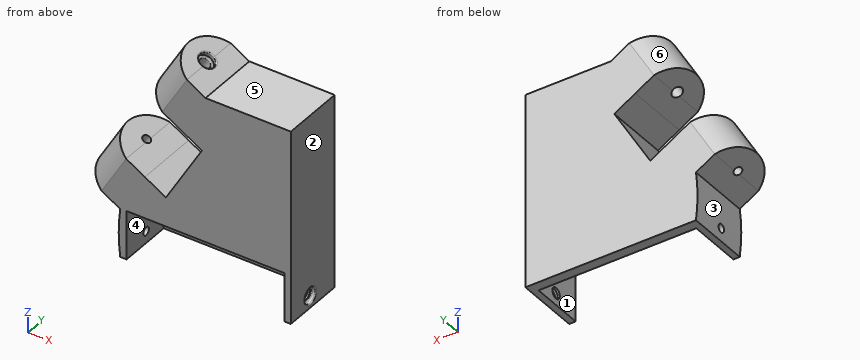
```python
from build123d import *

# Parameters (mm, degrees)
BOSS_EXTRUDE2_DEPTH                             = 29.972
EXTRUDE_THIN2_DEPTH                             = 29.972
BOSS_EXTRUDE3_DEPTH                             = 22.86
BOSS_EXTRUDE4_DEPTH                             = 22.86
SKETCH12_R                                      = 1.905
CUT_EXTRUDE2_DEPTH                              = 111.410659875
BOSS_EXTRUDE6_DEPTH                             = 29.972
CBORE_FOR_6_PAN_HEAD_MACHINE_SCREW1_D           = 3.7500052
CBORE_FOR_6_PAN_HEAD_MACHINE_SCREW1_CBORE_D     = 7.5000104
CBORE_FOR_6_PAN_HEAD_MACHINE_SCREW1_CBORE_DEPTH = 2.032
CUT_EXTRUDE4_REACH                              = 107.839
SKETCH18_R                                      = 2.5
FILLET1_R                                       = 0.5
SKETCH19_W                                      = 73.969126852
SKETCH19_H                                      = 25.4
CUT_EXTRUDE5_DEPTH                              = 22.86
CUT_EXTRUDE7_START                              = -80.649491
SKETCH21_R                                      = 1.905
CUT_EXTRUDE7_DEPTH                              = 80.649491
CBORE_FOR_6_PAN_HEAD_MACHINE_SCREW2_D           = 3.7500052
CBORE_FOR_6_PAN_HEAD_MACHINE_SCREW2_CBORE_D     = 7.5000104
CBORE_FOR_6_PAN_HEAD_MACHINE_SCREW2_CBORE_DEPTH = 2.032
SKETCH26_R                                      = 2.54
CUT_EXTRUDE9_DEPTH                              = 3.048
FILLET3_R                                       = 0.5
CUT_EXTRUDE11_DEPTH                             = 29.972


with BuildPart() as part:
    # Sketch1 → Boss-Extrude2 (new body)
    with BuildSketch(Plane(origin=(0, 0, 0), x_dir=(1, 0, 0), z_dir=(0, 1, 0))):
        Polygon((-40.005, 45.466), (-40.005, 22.86), (0, -45.466), (40.005, -45.466), (40.005, 45.466), align=None)
    extrude(amount=BOSS_EXTRUDE2_DEPTH)

    # Sketch8 → Extrude-Thin2 (add)
    with BuildSketch(Plane(origin=(0, 0, 0), x_dir=(1, 0, 0), z_dir=(0, 1, 0))):
        Polygon((-40.005, 22.86), (-28.454605215, 3.132659066), (-37.222312297, -2.000849727), (-48.772707082, 17.726491207), align=None)
        Polygon((-11.550394785, -25.738659066), (0, -45.466), (-8.767707082, -50.599508793), (-20.318101866, -30.872167859), align=None)
    extrude(amount=EXTRUDE_THIN2_DEPTH)

    # Sketch10 → Boss-Extrude3 (add)
    with BuildSketch(Plane(origin=(19.824382752, 0, 33.85878705), x_dir=(0.862963295, 0, -0.505266614), z_dir=(0.505266614, 0, 0.862963295))):
        with BuildLine():
            Line((-33.132451849, 29.972), (-33.132451849, 0))
            ThreePointArc((-33.132451849, 0), (-44.041101893, 14.986), (-33.132451849, 29.972))
        make_face()
    extrude(amount=-BOSS_EXTRUDE3_DEPTH)

    # Sketch11 → Boss-Extrude4 (add)
    with BuildSketch(Plane(origin=(-8.630222463, 0, -14.739872016), x_dir=(0.862963295, 0, -0.505266614), z_dir=(0.505266614, 0, 0.862963295))):
        with BuildLine():
            Line((-33.132451849, 0), (-33.132451849, 29.972))
            ThreePointArc((-33.132451849, 29.972), (-44.041101893, 14.986), (-33.132451849, 0))
        make_face()
    extrude(amount=-BOSS_EXTRUDE4_DEPTH)

    # Sketch12 → Cut-Extrude2 (cut, through all)
    with BuildSketch(Plane(origin=(21.107759951, 0, 36.050713821), x_dir=(0.862963295, 0, -0.505266614), z_dir=(0.505266614, 0, 0.862963295))):
        with Locations((-33.881101893, 14.986)):
            Circle(SKETCH12_R)
    extrude(amount=-CUT_EXTRUDE2_DEPTH, mode=Mode.SUBTRACT)

    # Sketch15 → Boss-Extrude6 (add)
    with BuildSketch(Plane(origin=(0, 29.972, 0), x_dir=(1, 0, 0), z_dir=(0, 1, 0))):
        with BuildLine():
            Line((-40.005, 45.466), (-40.005, 22.86))
            ThreePointArc((-40.005, 22.86), (-40.726132774, 34.163), (-40.005, 45.466))
        make_face()
    extrude(amount=-BOSS_EXTRUDE6_DEPTH)

    # CBORE for #6 Pan Head Machine Screw1 (through all)
    with Locations(Plane(origin=(19.824382752, 0, 33.85878705), x_dir=(0.862963295, 0, -0.505266614), z_dir=(0.505266614, 0, 0.862963295))):
        with Locations((-33.881101893, 14.986)):
            CounterBoreHole(CBORE_FOR_6_PAN_HEAD_MACHINE_SCREW1_D / 2, CBORE_FOR_6_PAN_HEAD_MACHINE_SCREW1_CBORE_D / 2, CBORE_FOR_6_PAN_HEAD_MACHINE_SCREW1_CBORE_DEPTH)

    # Sketch18 → Cut-Extrude4 (cut, up to next)
    with BuildSketch(Plane(origin=(18.797680994, 0, 32.105245634), x_dir=(0.862963295, 0, -0.505266614), z_dir=(0.505266614, 0, 0.862963295)), mode=Mode.PRIVATE) as cut_extrude4_sk1:
        with Locations((-33.881101893, 14.986)):
            Circle(SKETCH18_R)
    cut_extrude4_tool1 = extrude(cut_extrude4_sk1.sketch, amount=-CUT_EXTRUDE4_REACH, mode=Mode.PRIVATE) & part.part
    add(cut_extrude4_tool1.solids().sort_by_distance((-10.440466, 14.986, 49.224235))[0], mode=Mode.SUBTRACT)

    # Fillet1
    fillet1_edges = [part.edges().sort_by_distance(p)[0] for p in [
        (-12.649881436, 14.986, 52.872529093),
        (-12.597874588, 14.986, 50.487401783),
    ]]
    fillet(fillet1_edges, radius=FILLET1_R)

    # Sketch19 → Cut-Extrude5 (cut)
    with BuildSketch(Plane(origin=(0, 0, -45.466), x_dir=(-1, 0, 0), z_dir=(0, 0, -1))):
        with Locations((0.027563426, 12.7)):
            Rectangle(SKETCH19_W, SKETCH19_H)
    extrude(amount=-CUT_EXTRUDE5_DEPTH, mode=Mode.SUBTRACT)

    # Sketch21 → Cut-Extrude7 (cut)
    with BuildSketch(Plane(origin=(40.005, 0, 0), x_dir=(0, 0, -1), z_dir=(1, 0, 0)).offset(CUT_EXTRUDE7_START)):
        with Locations((39.878, 13.391837379)):
            Circle(SKETCH21_R)
    extrude(amount=CUT_EXTRUDE7_DEPTH, mode=Mode.SUBTRACT)

    # CBORE for #6 Pan Head Machine Screw2 (through all)
    with Locations(Plane(origin=(40.005, 0, 0), x_dir=(0, 0, -1), z_dir=(1, 0, 0))):
        with Locations((39.878, 13.391837379)):
            CounterBoreHole(CBORE_FOR_6_PAN_HEAD_MACHINE_SCREW2_D / 2, CBORE_FOR_6_PAN_HEAD_MACHINE_SCREW2_CBORE_D / 2, CBORE_FOR_6_PAN_HEAD_MACHINE_SCREW2_CBORE_DEPTH)

    # Sketch26 → Cut-Extrude9 (cut)
    with BuildSketch(Plane(origin=(40.005, 0, 0), x_dir=(0, 0, -1), z_dir=(1, 0, 0))):
        with Locations(Location((39.878, 13.391837379, 0), (0, 0, 180))):  # turned: the seam where the file's is
            Circle(SKETCH26_R)
    extrude(amount=-CUT_EXTRUDE9_DEPTH, mode=Mode.SUBTRACT)

    # Fillet3
    fillet3_edges = [part.edges().sort_by_distance(p)[0] for p in [
        (40.005, 13.391837379, -36.1279948),
        (37.973, 13.391837379, -36.1279948),
    ]]
    fillet(fillet3_edges, radius=FILLET3_R)

    # Sketch28 → Cut-Extrude11 (cut)
    with BuildSketch(Plane(origin=(0, 29.972, 0), x_dir=(1, 0, 0), z_dir=(0, 1, 0))):
        Polygon((-11.550394785, -25.738659066), (-1.686724318, -19.963461674), (-18.590934748, 8.907856459), (-28.454605215, 3.132659066), align=None)
    extrude(amount=-CUT_EXTRUDE11_DEPTH, mode=Mode.SUBTRACT)


solid = part.part
```
The listing builds one solid part. Answer for the finished solid, in the listing's coordinates (mm). Face numbers are marked on the shaded views. A direction names the side the tool comes from. Give positions to 0.01 mm unless a question says otherwise; leave off trailing zeros. Order: outer loops, then holes, each group sorted by start corner. A loop starts at its lowest first (then second) coordinate and runs counter-clockwise, first axis right, second up. Notation, with made-up numbers: (78.5, 55.25) -> (96.5, 55.25) arc R30 ccw to (96.5, 84.25) -> close; hole circle Ø10 at (18.25, 1). An arc over 180 degrees is marked (long way). Answer as a JSON object with one key per item and string values. Group by question number.
Item 1: The part is cut by section C-C on y = 6.75. Write down the section's boundary in (x, z) (1 decimal), and give its area (3 significant figures).
Item 2: Flat-ended cylindrical pins translate along their axes: pin 1 (5 mm diameter, centred on y = 13.39, z = -39.88, fed in from +X); pin 2 (7 mm diameter, centred on y = 14, z = -40, fed in from +X); pin 3 (10 mm diameter, centred on y = 13.39, z = -39.88, fed in from -X). Find the tip coordinate at first contact, or state that the pin passes through.
Item 3: Consider L1, parallel to X at y = 24.5, z = -37.5 (3 decimals); L2, parallel to Z at x = 23, y = 7.25; L3, parallel to Y at x = 0.5, z = -38. Determine where each line is inside the solid, lowest interval first. Write a range as from..to.
Item 4: The part is cut by section B-B on z = -25. Write down the section's boundary in (x, y) (3 decimals), and give its area (3 significant figures).
Item 5: Determine the mould class of the marked faces 1, 2 and 3 for opening direction X: pulls with the +X half, pulls with the -X half, needs draft (parallel to the pull), parting line crosses it, or undercut.
Item 6: A tool of negligible diameter and unlimited length cuts with its end or side. For the marked faces 4, 5 and 6, from which of +Z, -Z, +X, -X, +Y, -Y can it reach the whole face along a straight path? Write none if from no direction.
Item 7: The part is cut by section A-A on x = 15. Write down the section's boundary in (y, z).
Item 8: The part is cut by section D-D on y = 23. Write down the section's boundary in (x, z) (1 decimal), and give its area (3 significant figures).
Result set:
{
 "1": {"outline": "(-56.2, -13.4) -> (-40, -22.9) arc R88.9 ccw to (-40, -45.5) -> (-37, -45.5) -> (-37, -22.6) -> (37, -22.6) -> (37, -45.5) -> (40, -45.5) -> (40, 45.5) -> (0, 45.5) -> (-16.2, 54.9) -> (-27.7, 35.2) -> (-1.7, 20) -> (-18.6, -8.9) -> (-44.6, 6.3) -> close", "area": "4,700 mm²"},
 "2": {"pin 1": "x = -37.01", "pin 2": "x = 39.99", "pin 3": "x = -40.72"},
 "3": {"L1": "-40.664..-37.012, 36.957..40.005", "L2": "-22.61..45.47", "L3": "25.4..29.97"},
 "4": {"outline": "(-40.253, 0) -> (-37.012, 0) -> (-37.012, 25.4) -> (36.957, 25.4) -> (36.957, 0) -> (40.005, 0) -> (40.005, 29.972) -> (-40.253, 29.972) -> close", "area": "527 mm²"},
 "5": {"face 1": "undercut", "face 2": "pulls with the +X half", "face 3": "pulls with the -X half"},
 "6": {"face 4": "-Z, -Y", "face 5": "+Z, +X, +Y, -Y", "face 6": "+Z, -X"},
 "7": {"outline": "(0, -22.61) -> (25.4, -22.61) -> (25.4, -45.47) -> (29.97, -45.47) -> (29.97, 45.47) -> (0, 45.47) -> close"},
 "8": {"outline": "(-56.3, -13.3) -> (-40, -22.9) arc R88.9 ccw to (-40, -45.5) -> (-37, -45.5) -> (-37, -22.6) -> (37, -22.6) -> (37, -45.5) -> (40, -45.5) -> (40, 45.5) -> (0, 45.5) -> (-16.3, 55) -> (-27.8, 35.3) -> (-1.7, 20) -> (-18.6, -8.9) -> (-44.7, 6.4) -> close", "area": "4,710 mm²"}
}
